```python
from build123d import *

# Parameters (mm, degrees)
SKETCH1_W                    = 30
SKETCH1_H                    = 30
BASE_FLANGE1_DEPTH           = 2
EDGE_FLANGE1_STRIP_W         = 10
EDGE_FLANGE1_STRIP_H         = 2
EDGE_FLANGE1_STRIP_CUT_DEPTH = 30
EDGE_FLANGE1_DEPTH           = 30


# Sheet-metal steps are written as plain solids
with BuildPart() as part:
    # Sketch1 → Base-Flange1 (new body)
    with BuildSketch(Plane(origin=(0, 0, 0), x_dir=(1, 0, 0), z_dir=(0, 1, 0))):
        Rectangle(SKETCH1_W, SKETCH1_H)
        with BuildLine():
            Line((-6.75, -6), (-6.75, 6))
            ThreePointArc((-6.75, 6), (-5, 7.75), (-3.25, 6))
            Line((-3.25, 6), (-3.25, -6))
            ThreePointArc((-3.25, -6), (-5, -7.75), (-6.75, -6))
        make_face(mode=Mode.SUBTRACT)
        with BuildLine():
            Line((3.25, -6), (3.25, 6))
            ThreePointArc((3.25, 6), (5, 7.75), (6.75, 6))
            Line((6.75, 6), (6.75, -6))
            ThreePointArc((6.75, -6), (5, -7.75), (3.25, -6))
        make_face(mode=Mode.SUBTRACT)
    extrude(amount=-BASE_FLANGE1_DEPTH)

    # Edge-Flange1 strip (across the edge) → Edge-Flange1 strip cut (cut)
    with BuildSketch(Plane(origin=(-15, 0, 15), x_dir=(0, 0, -1), z_dir=(1, 0, 0))):
        with Locations((-4, -1)):
            Rectangle(EDGE_FLANGE1_STRIP_W, EDGE_FLANGE1_STRIP_H)
    extrude(amount=EDGE_FLANGE1_STRIP_CUT_DEPTH, mode=Mode.SUBTRACT)

    # Edge-Flange1 section (across the edge) → Edge-Flange1 (add)
    with BuildSketch(Plane(origin=(-15, 0, 15), x_dir=(0, 0, -1), z_dir=(1, 0, 0))):
        with BuildLine():
            Line((-2, 1), (-2, 28))
            Line((-2, 28), (0, 28))
            Line((0, 28), (0, 1))
            ThreePointArc((0, 1), (0.292893219, 0.292893219), (1, 0))
            Line((1, 0), (1, -2))
            ThreePointArc((1, -2), (-1.121320344, -1.121320344), (-2, 1))
        make_face()
    extrude(amount=EDGE_FLANGE1_DEPTH)


solid = part.part
```
Read the model definition and answer for the solid it produces. Units are mm, in the model's axes. A direction names the side the tool comes from. Give positions to 0.01 mm unless a question says otherwise; leave off trailing zeros. Order: outer loops, then holes, each group sorted by start corner. A loop starts at its lowest first (then second) coordinate and runs counter-clockwise, first axis right, second up. Notation, with made-up numbers: (70.25, -38) -> (126.25, -38) arc R30 cw to (126.25, -1) -> close; hole circle Ø9 at (-16.5, 46). An arc over 180 degrees is marked (long way). Write item = value, one per line.
1. A cutting plane is placed at B-B, the plane z = 3.5. Write down the section's boundary in (x, y), and give its area (3 significant figures).
Numbers:
outline = (-15, -2) -> (-6.75, -2) -> (-6.75, 0) -> (-15, 0) -> close; (-3.25, -2) -> (3.25, -2) -> (3.25, 0) -> (-3.25, 0) -> close; (6.75, -2) -> (15, -2) -> (15, 0) -> (6.75, 0) -> close
area = 46.0 mm²
2. Straight lines are drawn through the part: line 1 along Z through (x, y) = (-13, 24.25); line 2 along Y through (x, z) = (7.25, 5); line 3 along Z through (x, y) = (-1.25, -0.75). For each, find the intervals that lie inside material, in ascending order.
Numbers:
line_1 = 15 to 17
line_2 = -2 to 0
line_3 = -15 to 16.44
3. Given pin 1 (3 mm diameter, centred on x = -0.5, z = 12, fed in from +Y); pin 2 (6 mm diameter, centred on x = 11.5, y = 8, fed in from -Z); pin 3 (12 mm diameter, centred on y = 5, z = -1.5, fed in from +X); pin 4 (1.5 mm diameter, centred on x = -4.5, z = -2, fed in from +Y), each flat-ended and moving along its own axis, determine where each tip first touches the part or whether it passes through.
Numbers:
pin_1 = 0
pin_2 = 15
pin_3 = 15
pin_4 = through
4. For faces 4 (the face through (5.04, -0.99, 7.75)), 5 (the face through (0, 14, 17)), 6 (the face through (0, 0, -1)), determine the directions among +Z, -Z, +X, -X, +Y, -Y from which every point of the face is accessible in a straight line to the end or side of a thin tool.
Numbers:
face_4 = +Y, -Y
face_5 = +Z, +X, -X, +Y, -Y
face_6 = -Z, +X, -X, +Y
5. The mould has two halves that part along X. Classify faces 1 (the face through (-15, -0.3, 6.9)), 2 (the face through (0, -1, -15)), 3 (the face through (4.96, -0.99, -7.75)): +X half, -X half, draft (parallel to the pull), parting line (faces both ways), or undercut.
Numbers:
face_1 = -X half
face_2 = draft
face_3 = undercut
6. A cutting plane is placed at A-A, the plane x = -5. Write down the section's boundary in (y, z).
Numbers:
outline = (-2, -15) -> (0, -15) -> (0, -7.75) -> (-2, -7.75) -> close; (-2, 7.75) -> (0, 7.75) -> (0, 14) arc R1 cw to (1, 15) -> (28, 15) -> (28, 17) -> (1, 17) arc R3 ccw to (-2, 14) -> close
7. A cutting plane is placed at C-C, the plane x = -1.25. Write down the section's boundary in (y, z).
Numbers:
outline = (-2, -15) -> (0, -15) -> (0, 14) arc R1 cw to (1, 15) -> (28, 15) -> (28, 17) -> (1, 17) arc R3 ccw to (-2, 14) -> close
8. A cutting plane is placed at D-D, the plane y = 8.75. Write down the section's boundary in (x, z).
Numbers:
outline = (-15, 15) -> (15, 15) -> (15, 17) -> (-15, 17) -> close
